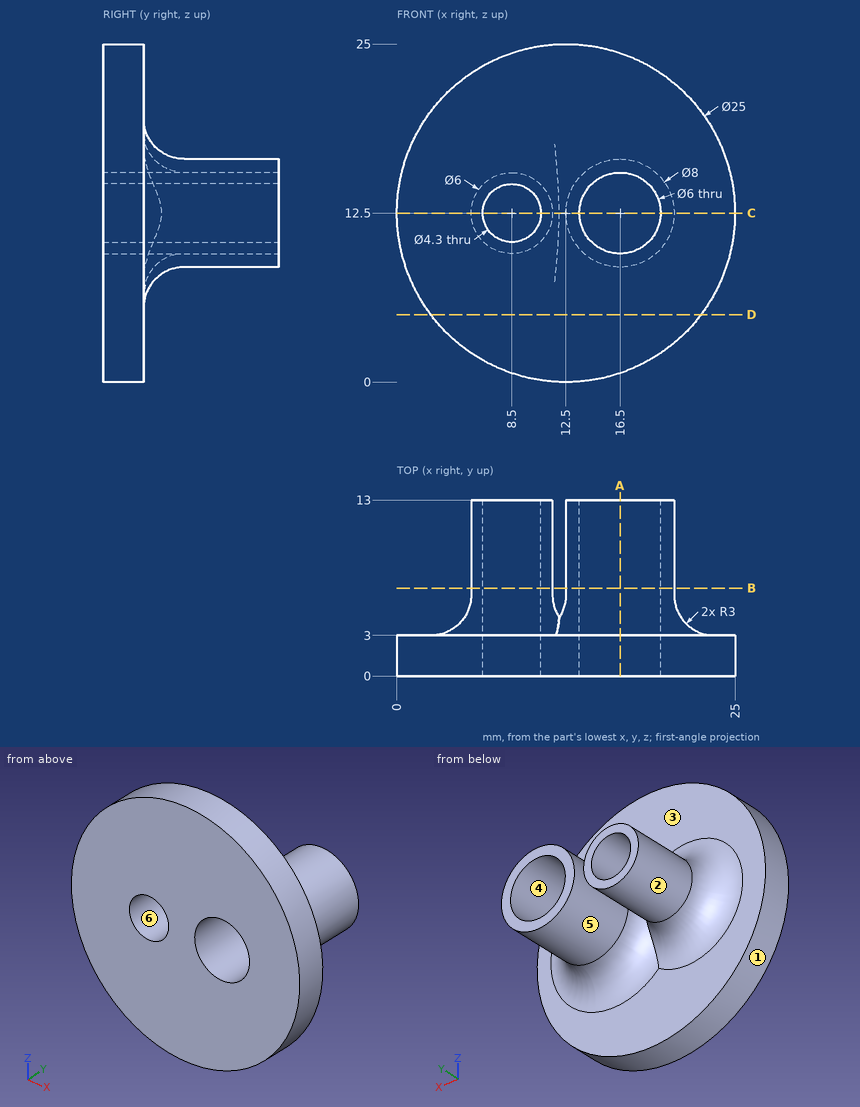
For this review, use the dimensioned drawing (mm, ordinates from the lowest corner) and the shaded views. A direction names the side the tool comes from. Round coordinates to 2 decimals unless told otherwise and drop trailing zeros. Loops run counter-clockwise (first coordinate to the right, second up) from the corner with the lowest first, then second, coordinate; pieces in that order, holes last. Notation, with made-up numbers: (5, -15) -> (22, -15) arc R31 cw to (22, 17) -> close; hole circle Ø11 at (50.5, 79.25). An arc over 180 degrees is marked (long way). Write item = value, one per line. Start each with the question number.
Item 1: Take a section at B-B on y = 6.5. Give the boundary of the cut face in (x, z).
Item 2: Insertion check: pin 1 (4 mm diameter, centred on x = 4, y = 9.5, fed in from +Z); pin 2 (2 mm diameter, centred on y = 4.5, z = 9, fed in from -X); pin 3 (1.5 mm diameter, centred on x = 14.5, y = 8, fed in from +Z); pin 4 (2.5 mm diameter, centred on x = 8.5, z = 12.5, fed in from +Y). Each pin has a flat end and moves straight along its axis. Give the tip position at first contact, or say it passes through.
Item 3: Take a section at C-C on z = 12.5. Give the boundary of the cut face in (x, y).
Item 4: Take a section at A-A on x = 16.5. Give the boundary of the cut face in (y, z).
Item 5: Mouldability with a two-part tool opening along Z and no side actions: class the marked faces 3, 4, 5 and 6 as released by +Z, released by -Z, zero draft, split by the parting line, or undercut.
Item 6: To check wall thickness, follow L1, parallel to X at y = 8, z = 12.5; L2, parallel to X at y = 8, z = 13.5; L3, parallel to X at y = 3.75, z = 12.5. State the ranges of each line that lie inside material, in increasing order.
Item 7: Take a section at D-D on z = 5. Give the boundary of the cut face in (x, y), plus the area to 3 significant figures.
Item 8: For the marked faces 1 and 2, list the 3-axis set-ups (+Z, -Z, +X, -X, +Y, -Y) from which the entire face can be reached by the end or side of a thin tool; tool diameter is ignored.
Result:
q1.outline = circle Ø6 at (8.5, 12.5); circle Ø8 at (16.5, 12.5); hole circle Ø4.3 at (8.5, 12.5); hole circle Ø6 at (16.5, 12.5)
q2.pin_1 = 14.16
q2.pin_2 = 5.62
q2.pin_3 = 16.3
q2.pin_4 = through
q3.outline = (0, 0) -> (6.35, 0) -> (6.35, 13) -> (5.5, 13) -> (5.5, 6) arc R3 cw to (2.5, 3) -> (0, 3) -> close; (10.65, 0) -> (13.5, 0) -> (13.5, 13) -> (12.5, 13) -> (12.5, 6) arc R3 cw to (12, 4.34) arc R3 cw to (11.5, 6) -> (11.5, 13) -> (10.65, 13) -> close; (19.5, 0) -> (25, 0) -> (25, 3) -> (23.5, 3) arc R3 cw to (20.5, 6) -> (20.5, 13) -> (19.5, 13) -> close
q4.outline = (0, 0.66) -> (3, 0.66) -> (3, 5.5) arc R3 cw to (6, 8.5) -> (13, 8.5) -> (13, 9.5) -> (0, 9.5) -> close; (0, 15.5) -> (13, 15.5) -> (13, 16.5) -> (6, 16.5) arc R3 cw to (3, 19.5) -> (3, 24.34) -> (0, 24.34) -> close
q5.face_3 = zero draft
q5.face_4 = undercut
q5.face_5 = split by the parting line
q5.face_6 = undercut
q6.L1 = 5.5 to 6.35, 10.65 to 11.5, 12.5 to 13.5, 19.5 to 20.5
q6.L2 = 5.67 to 6.6, 10.4 to 11.33, 12.63 to 13.67, 19.33 to 20.37
q6.L3 = 4.48 to 6.35, 10.65 to 13.5, 19.5 to 21.52
q7.outline = (2.5, 0) -> (22.5, 0) -> (22.5, 3) -> (2.5, 3) -> close
q7.area = 60.0 mm²
q8.face_1 = +Y, -Y
q8.face_2 = +Y
